Verification items for the finished model (mm, model axes). A direction names the side the tool comes from. Round coordinates to 2 decimals unless told otherwise and drop trailing zeros. Loops run counter-clockwise (first coordinate to the right, second up) from the corner with the lowest first, then second, coordinate; pieces in that order, holes last. Notation, with made-up numbers: (23, 49.5) - (59, 49.5) arc R27 ccw to (59, 66.5) - close; hole circle Ø10 at (30.25, -24). An arc over 180 degrees is marked (long way). Use a Markdown table: item, result. Add a question column.
```python
from build123d import *

# Parameters (mm, degrees)
EXTRUDE_1_DEPTH     = 7.75
SKETCH_3_R          = 1
SKETCH_3_W          = 12
SKETCH_3_H          = 23
CUT_EXTRUDE_1_DEPTH = 34.594084301
CHAMFER_1_SIZE      = 2


with BuildPart() as part:
    # 草圖2 → 填料-伸長1 (new, symmetric)
    with BuildSketch(Plane(origin=(0, 0, 0), x_dir=(0, 0, -1), z_dir=(1, 0, 0))):
        Polygon((27.75, 3.5), (32.5, 3.5), (32.5, 0), (0, 0), (0, 3.5), (4.75, 3.5), (4.75, 2.5), (27.75, 2.5), align=None)
    extrude(amount=EXTRUDE_1_DEPTH, both=True)

    # 草圖3 → 除料-伸長1 (cut, through all)
    with BuildSketch(Plane.XZ):
        with Locations(Location((0, -2, 0), (0, 0, 270))):
            Circle(SKETCH_3_R)
        with Locations(Location((0, -30.5, 0), (0, 0, 270))):
            Circle(SKETCH_3_R)
        with Locations((0, -16.25)):
            Rectangle(SKETCH_3_W, SKETCH_3_H)
    extrude(amount=-CUT_EXTRUDE_1_DEPTH, mode=Mode.SUBTRACT)

    # 導角1
    chamfer_1_edges = [part.edges().sort_by_distance(p)[0] for p in [
        (7.75, 1.75, -32.5),
        (-7.75, 1.75, 0),
        (7.75, 1.75, 0),
        (-7.75, 1.75, -32.5),
    ]]
    chamfer(chamfer_1_edges, length=CHAMFER_1_SIZE)


solid = part.part
```
Q1. Go/stop test with flat-tipped pins: pin 1 Ø0.9 at (x, z) = (7.5, -22) entering from +Y; pin 2 Ø6 at (x, z) = (-2, -24.5) entering from -Y. Record where each tip stops, or that it passes through.
Q2. Release check for a two-part mould opening along X. For faces 4 (the face through (-6, 1, -16)), 5 (the face through (-7.75, 1, -16)), 6 (the face through (0, 3.5, -29)), 7 (the face through (6.74, 1.77, -31.51)) record: +X half, -X half, draft (parallel to the pull), parting line (faces both ways), or undercut.
Q3. Section check D-D on x = -4. Record the cut outline in (y, z).
Q4. Set-up check for faces 1 (the face through (7.75, 1, -16)), 2 (the face through (7, 2.5, -16)), 3 (the face through (6, 1, -16)): record each of +Z, -Z, +X, -X, +Y, -Y from which the full face is reachable in a straight line by a thin tool's end or side.
Q5. Section check B-B on z = -20.5. Record the cut outline in (x, y), plus the area to 3 significant figures.
Q6. Section check C-C on y = 1. Record the cut outline in (x, z), plus the area to 3 significant figures.
Q7. Section check A-A on x = 0. Record the cut outline in (y, z).
Q8. Thickness scan on line 1 along Z through (x, y) = (3, 3.2); line 2 along X through (y, z) = (2.05, -13.5); line 3 along X through (y, z) = (1.05, -2). Record the ranges inside material, lowest first.
Determined:
| question | item | result |
|---|---|---|
| 1 | pin 1 | stops at y = 2.5 |
| 1 | pin 2 | passes through |
| 2 | face 4 | undercut |
| 2 | face 5 | -X half |
| 2 | face 6 | draft |
| 2 | face 7 | +X half |
| 3 | outline | (0, -32.5) - (3.5, -32.5) - (3.5, -27.75) - (0, -27.75) - close; (0, -4.75) - (3.5, -4.75) - (3.5, 0) - (0, 0) - close |
| 4 | face 1 | +Z, -Z, +X, +Y, -Y |
| 4 | face 2 | +X, -X, +Y |
| 4 | face 3 | +Y, -Y |
| 5 | outline | (-7.75, 0) - (-6, 0) - (-6, 2.5) - (-7.75, 2.5) - close; (6, 0) - (7.75, 0) - (7.75, 2.5) - (6, 2.5) - close |
| 5 | area | 8.75 mm² |
| 6 | outline | (-7.75, -30.5) - (-5.75, -32.5) - (5.75, -32.5) - (7.75, -30.5) - (7.75, -2) - (5.75, 0) - (-5.75, 0) - (-7.75, -2) - close; hole (-6, -27.75) - (6, -27.75) - (6, -4.75) - (-6, -4.75) - close; hole circle Ø2 at (0, -30.5); hole circle Ø2 at (0, -2) |
| 6 | area | 213 mm² |
| 7 | outline | (0, -32.5) - (3.5, -32.5) - (3.5, -31.5) - (0, -31.5) - close; (0, -29.5) - (3.5, -29.5) - (3.5, -27.75) - (0, -27.75) - close; (0, -4.75) - (3.5, -4.75) - (3.5, -3) - (0, -3) - close; (0, -1) - (3.5, -1) - (3.5, 0) - (0, 0) - close |
| 8 | line 1 | z = -32.5 to -27.75, -4.75 to 0 |
| 8 | line 2 | x = -7.75 to -6, 6 to 7.75 |
| 8 | line 3 | x = -7.75 to -1, 1 to 7.75 |
